```python
from build123d import *
from build123d.topology import SkipClean

# Parameters (mm, degrees)
SKETCH_2_R          = 1.288183927
SKETCH_2_R_2        = 0.75
CUT_EXTRUDE_1_DEPTH = 15.5
SKETCH_3_R          = 0.3
CUT_EXTRUDE_2_DEPTH = 4
SKETCH_8_W          = 0.393463538
SKETCH_8_H          = 2


with BuildPart() as part:
    # Sketch 1 → Revolve 1 (revolve)
    with SkipClean():  # the faces are left unmerged after this step: merging them gives an invalid solid
        with BuildSketch(Plane.XY, mode=Mode.PRIVATE) as revolve_1_sk:
            with BuildLine():
                Line((1, 15.4), (1, 0))
                Line((1, 0), (2, 0))
                Line((2, 0), (2, 15.7))
                add(Edge.make_bspline(
                    [(1, 15.4), (2, 15.4), (2, 15.7)],
                    knots=[4.71238898, 4.71238898, 4.71238898, 6.283185307, 6.283185307, 6.283185307], degree=2, weights=[1, 0.707106781, 1]))
            make_face()
            with BuildLine():
                add(Edge.make_bspline(
                    [(1, 16), (0, 16), (0, 15.7)],
                    knots=[1.570796327, 1.570796327, 1.570796327, 3.141592654, 3.141592654, 3.141592654], degree=2, weights=[1, 0.707106781, 1]))
                add(Edge.make_bspline(
                    [(0, 15.7), (0, 15.4), (1, 15.4)],
                    knots=[3.141592654, 3.141592654, 3.141592654, 4.71238898, 4.71238898, 4.71238898], degree=2, weights=[1, 0.707106781, 1]))
                Line((1, 15.4), (1, 16))
            make_face()
            with BuildLine():
                Line((1, 16), (1, 15.4))
                add(Edge.make_bspline(
                    [(1, 15.4), (2, 15.4), (2, 15.7)],
                    knots=[4.71238898, 4.71238898, 4.71238898, 6.283185307, 6.283185307, 6.283185307], degree=2, weights=[1, 0.707106781, 1]))
                add(Edge.make_bspline(
                    [(2, 15.7), (2, 16), (1, 16)],
                    knots=[0, 0, 0, 1.570796327, 1.570796327, 1.570796327], degree=2, weights=[1, 0.707106781, 1]))
            make_face()
        revolve(revolve_1_sk.sketch.rotate(Axis((1, 22.010661338, 0), (0, -1, 0)), 180), axis=Axis((1, 22.010661338, 0), (0, -1, 0)))
    add(part.part.scale(1), mode=Mode.REPLACE)  # the faces are merged on a copy

    # Sketch 2 → Cut-Extrude 1 (cut)
    with BuildSketch(Plane.XZ):
        with Locations((1, 0)):
            Circle(SKETCH_2_R)
        with Locations((1, 0)):
            Circle(SKETCH_2_R_2, mode=Mode.SUBTRACT)
    extrude(amount=-CUT_EXTRUDE_1_DEPTH, mode=Mode.SUBTRACT)

    # Sketch 3 → Cut-Extrude 2 (cut)
    with BuildSketch(Plane(origin=(0, 0, 0), x_dir=(-1, 0, 0), z_dir=(0, -1, 0))):
        with Locations(Location((-1, 0, 0), (0, 0, 180))):
            Circle(SKETCH_3_R)
    extrude(amount=-CUT_EXTRUDE_2_DEPTH, mode=Mode.SUBTRACT)

    # Sketch 8 → Cut-Revolve 1 (revolve, cut)
    with BuildSketch(Plane.XY, mode=Mode.PRIVATE) as cut_revolve_1_sk:
        with Locations((1.746731769, 13)):
            Rectangle(SKETCH_8_W, SKETCH_8_H)
        with Locations((1.746731769, 9)):
            Rectangle(SKETCH_8_W, SKETCH_8_H)
    revolve(cut_revolve_1_sk.sketch.rotate(Axis((1, 0, 0), (0, 1, 0)), 90), axis=Axis((1, 0, 0), (0, 1, 0)), mode=Mode.SUBTRACT)


solid = part.part
```
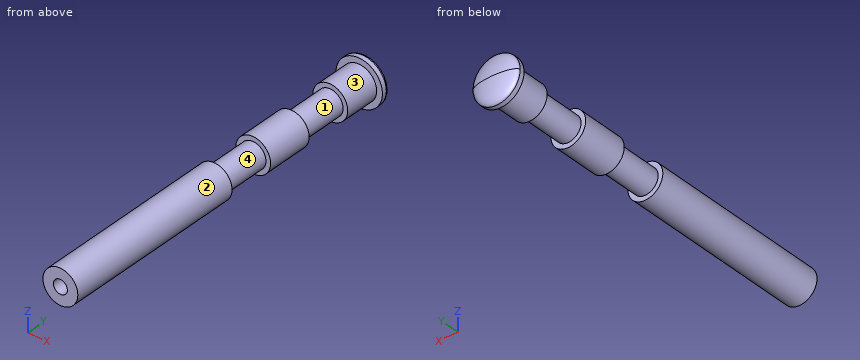
Input: part model. Units: mm. Frame: model coordinates. Face numbers are marked on the shaded views. A direction names the side the tool comes from. Round coordinates to 2 decimals unless told otherwise and drop trailing zeros. Write each loop counter-clockwise with the first axis right and the second up, starting at its lowest first coordinate (ties: lowest second). Pieces come first, ordered by that corner, then holes. Notation, with made-up numbers: (17, 75.25) - (27, 75.25) arc R23 cw to (27, 99.25) - close; hole circle Ø6 at (50, 85.5). An arc over 180 degrees is marked (long way). Write item = value, one per line.
(1) Material intervals for probe 1 along Z at (x, y) = (1, 1.15); probe 2 along Y at (x, z) = (1.3, -0.65); probe 3 along X at (y, z) = (8.75, -0.1), sorted ascending.
Geometry check:
probe_1 = -0.75 to -0.3, 0.3 to 0.75
probe_2 = 0 to 8, 10 to 12, 14 to 15.91
probe_3 = 0.46 to 1.54
(2) Pull-direction query (Y, two-part tool) for the marked faces 1 and 2; classes: +Y half, -Y half, draft (parallel to the pull), parting line (faces both ways), or undercut.
Geometry check:
face_1 = undercut
face_2 = draft
(3) Access query for the marked faces 3 and 4. Directions: +Z, -Z, +X, -X, +Y, -Y. A direction counts if a zero-diameter tool reaches every point of the face in a straight line with its end or side. Return the directions, or none.
Geometry check:
face_3 = -Y
face_4 = none
(4) Section query A-A on y = 2.75. Output: boundary loops of the cut face in (x, z), then the cut area to 3 significant figures.
Geometry check:
outline = circle Ø1.5 at (1, 0); hole circle Ø0.6 at (1, 0)
area = 1.48 mm^2
(5) Section query B-B on y = 10.25. Output: boundary loops of the cut face in (x, z), then the cut area to 3 significant figures.
Geometry check:
outline = circle Ø1.5 at (1, 0)
area = 1.77 mm^2
